from build123d import *

# Parameters (mm, degrees)
F0_W     = 190.5
F0_H     = 38.1
F1_DEPTH = 6.35


with BuildPart() as f1:
    # F0 (on Front) → F1 (new body)
    with BuildSketch(Plane.XZ):
        with BuildLine():
            Line((-70.64375, 21.040363), (-70.64375, -23.409637))
            Line((-70.64375, -23.409637), (119.85625, -23.409637))
            Line((119.85625, -23.409637), (119.85625, 21.040363))
            Line((119.85625, 21.040363), (119.85625, 71.840363))
            Line((119.85625, 71.840363), (95.5675, 71.840363))
            Line((95.5675, 71.840363), (90.4875, 21.040363))
            Line((90.4875, 21.040363), (87.3125, -10.709637))
            ThreePointArc((87.3125, -10.709637), (81.75625, -16.265887), (76.2, -10.709637))
            Line((76.2, -10.709637), (73.025, 21.040363))
            Line((73.025, 21.040363), (67.945, 71.840363))
            Line((67.945, 71.840363), (57.4675, 71.840363))
            Line((57.4675, 71.840363), (52.3875, 21.040363))
            Line((52.3875, 21.040363), (49.2125, -10.709637))
            ThreePointArc((49.2125, -10.709637), (43.65625, -16.265887), (38.1, -10.709637))
            Line((38.1, -10.709637), (34.925, 21.040363))
            Line((34.925, 21.040363), (29.845, 71.840363))
            Line((29.845, 71.840363), (19.3675, 71.840363))
            Line((19.3675, 71.840363), (14.2875, 21.040363))
            Line((14.2875, 21.040363), (11.1125, -10.709637))
            ThreePointArc((11.1125, -10.709637), (5.55625, -16.265887), (0, -10.709637))
            Line((0, -10.709637), (-3.175, 21.040363))
            Line((-3.175, 21.040363), (-8.255, 71.840363))
            Line((-8.255, 71.840363), (-18.7325, 71.840363))
            Line((-18.7325, 71.840363), (-23.8125, 21.040363))
            Line((-23.8125, 21.040363), (-26.9875, -10.709637))
            ThreePointArc((-26.9875, -10.709637), (-32.54375, -16.265887), (-38.1, -10.709637))
            Line((-38.1, -10.709637), (-41.275, 21.040363))
            Line((-41.275, 21.040363), (-46.355, 71.840363))
            Line((-46.355, 71.840363), (-70.64375, 71.840363))
            Line((-70.64375, 71.840363), (-70.64375, 21.040363))
        make_face()
        with Locations((24.60625, -42.459637)):
            Rectangle(F0_W, F0_H)
    extrude(amount=F1_DEPTH)


solid = f1.part
For this review, take the finished solid that the model builds, in its own axes (mm). A direction names the side the tool comes from. Round coordinates to 2 decimals unless told otherwise and drop trailing zeros. Write each loop counter-clockwise with the first axis right and the second up, starting at its lowest first coordinate (ties: lowest second). Pieces come first, ordered by that corner, then holes. Notation, with made-up numbers: (32.5, 40) - (74.5, 40) arc R32 cw to (74.5, 66) - close; hole circle Ø11 at (-38.75, 0.25). An arc over 180 degrees is marked (long way). Use a Markdown table: item, result.
Q1. Wall thickness on line 1 along X through (y, z) = (-1.5, 45); line 2 along X through (y, z) = (-0.5, 66); line 3 along Z through (x, y) = (45, -0.75): over which ranges is each line inside the solid? List them lowest first.
Derived:
| item | result |
|---|---|
| line 1 | x = -70.64 to -43.67, -21.42 to -5.57, 16.68 to 32.53, 54.78 to 70.63, 92.88 to 119.86 |
| line 2 | x = -70.64 to -45.77, -19.32 to -7.67, 18.78 to 30.43, 56.88 to 68.53, 94.98 to 119.86 |
| line 3 | z = -61.51 to -16.1 |
Q2. We need section D-D (x = 45). Give the boundary of the cut face in (y, z), plus the area to 3 significant figures.
Derived:
| item | result |
|---|---|
| outline | (-6.35, -61.51) - (0, -61.51) - (0, -16.1) - (-6.35, -16.1) - close |
| area | 288 mm2 |
Q3. We need section C-C (z = 62). Give the boundary of the cut face in (x, y), plus the area to 3 significant figures.
Derived:
| item | result |
|---|---|
| outline | (-70.64, -6.35) - (-45.37, -6.35) - (-45.37, 0) - (-70.64, 0) - close; (-19.72, -6.35) - (-7.27, -6.35) - (-7.27, 0) - (-19.72, 0) - close; (18.38, -6.35) - (30.83, -6.35) - (30.83, 0) - (18.38, 0) - close; (56.48, -6.35) - (68.93, -6.35) - (68.93, 0) - (56.48, 0) - close; (94.58, -6.35) - (119.86, -6.35) - (119.86, 0) - (94.58, 0) - close |
| area | 558 mm2 |
Q4. We need section B-B (y = -4). Give the boundary of the cut face in (x, z) (1 decimal).
Derived:
| item | result |
|---|---|
| outline | (-70.6, -61.5) - (119.9, -61.5) - (119.9, 71.8) - (95.6, 71.8) - (87.3, -10.7) arc R5.6 cw to (76.2, -10.7) - (67.9, 71.8) - (57.5, 71.8) - (49.2, -10.7) arc R5.6 cw to (38.1, -10.7) - (29.8, 71.8) - (19.4, 71.8) - (11.1, -10.7) arc R5.6 cw to (0, -10.7) - (-8.3, 71.8) - (-18.7, 71.8) - (-27, -10.7) arc R5.6 cw to (-38.1, -10.7) - (-46.4, 71.8) - (-70.6, 71.8) - close |
Q5. We need section A-A (z = 6.5). Give the boundary of the cut face in (x, y), plus the area to 3 significant figures.
Derived:
| item | result |
|---|---|
| outline | (-70.64, -6.35) - (-39.82, -6.35) - (-39.82, 0) - (-70.64, 0) - close; (-25.27, -6.35) - (-1.72, -6.35) - (-1.72, 0) - (-25.27, 0) - close; (12.83, -6.35) - (36.38, -6.35) - (36.38, 0) - (12.83, 0) - close; (50.93, -6.35) - (74.48, -6.35) - (74.48, 0) - (50.93, 0) - close; (89.03, -6.35) - (119.86, -6.35) - (119.86, 0) - (89.03, 0) - close |
| area | 840 mm2 |
Q6. Machinability: for faces 1 (the flat face through (53.398, -3.131, 31.143)), 2 (the flat face through (23, -3, -61.51)), which of the approach directions +Z, -Z, +X, -X, +Y, -Y give a long, thin tool a straight path to every point of the face, cutting with its end or side? Answer none if there is none.
Derived:
| item | result |
|---|---|
| face 1 | +Z, +Y, -Y |
| face 2 | -Z, +X, -X, +Y, -Y |
